```python
from build123d import *

# Parameters (mm, degrees)
SZKIC1_W                    = 164.5
SZKIC1_H                    = 25.5
DODANIE_WYCI_GNI_CIE1_DEPTH = 1
SZKIC3_W                    = 160.5
SZKIC3_H                    = 21.5
SZKIC2_W                    = 164.5
SZKIC2_H                    = 25.5
SZKIC3_140_W                = 158.5
SZKIC3_140_H                = 19.5
SZKIC2_152_W                = 162.5
SZKIC2_152_H                = 23.5


with BuildPart() as part:
    # Szkic1 → Dodanie-wyciągnięcie1 (new body)
    with BuildSketch(Plane.XY):
        Rectangle(SZKIC1_W, SZKIC1_H)
    extrude(amount=DODANIE_WYCI_GNI_CIE1_DEPTH)

    # Szkic3 → Wyciągnięcie po profilach2 section 0
    with BuildSketch(Plane.XY.offset(5.5)):
        Rectangle(SZKIC3_W, SZKIC3_H)
    # Szkic2 → Wyciągnięcie po profilach2 section 1
    with BuildSketch(Plane.XY.offset(1)):
        Rectangle(SZKIC2_W, SZKIC2_H)
    loft()

    # Szkic3<140> → Wycięcie-wyciągnięcie po profilach1 section 0
    with BuildSketch(Plane.XY.offset(5.5)):
        Rectangle(SZKIC3_140_W, SZKIC3_140_H)
    # Szkic2<152> → Wycięcie-wyciągnięcie po profilach1 section 1
    with BuildSketch(Plane.XY.offset(1)):
        Rectangle(SZKIC2_152_W, SZKIC2_152_H)
    loft(mode=Mode.SUBTRACT)


solid = part.part
```
Geometry: final body of the model. Coordinates: model frame, mm. Round coordinates to 2 decimals unless told otherwise and drop trailing zeros. Use CSV: the item, a comma, the result in double quotes. Start each with the question number.
Q1. First-contact query: pin 1 (3 mm diameter, centred on x = 40.5, z = 4.5, fed in from +Y); pin 2 (2 mm diameter, centred on y = 5.5, z = 3.5, fed in from -X); pin 3 (7 mm diameter, centred on x = -40, y = -3.5, fed in from +Z). Flat tips, straight axial feed; report the tip coordinate or a pass-through.
Q2. Material intervals for line 1 along Z through (x, y) = (-13, -5); line 2 along Y through (x, z) = (73.5, 4); line 3 along Y through (x, z) = (-61, 4.5), sorted ascending. Write a range as from..to.
Q3. Mould query, pull axis Y, two halves, no side actions, for faces 1 (the face through (-5, -10, 5.5)), 2 (the face through (-1, 0, 1)). Classes: +Y half, -Y half, draft (parallel to the pull), parting line (faces both ways), or undercut.
Result set:
1,pin 1,"stops at y = 11.86"
1,pin 2,"stops at x = -81.58"
1,pin 3,"stops at z = 1"
2,line 1,"z = 0..1"
2,line 2,"y = -11.42..-10.42, 10.42..11.42"
2,line 3,"y = -11.19..-10.19, 10.19..11.19"
3,face 1,"draft"
3,face 2,"undercut"
